CAD build for the part. Positions are in the model's coordinates, mm. A direction names the side the tool comes from. Give positions to 0.01 mm unless a question says otherwise; leave off trailing zeros. Order: outer loops, then holes, each group sorted by start corner. A loop starts at its lowest first (then second) coordinate and runs counter-clockwise, first axis right, second up.
```python
from build123d import *

# Parameters (mm, degrees)
BOSS_EXTRUDE1_DEPTH = 2
SKETCH2_R           = 0.74
CUT_EXTRUDE1_DEPTH  = 5.6
SKETCH6_W           = 79.5
SKETCH6_H           = 15
SKETCH6_R           = 3.2
CUT_EXTRUDE3_DEPTH  = 1.2
SKETCH7_R           = 3.2
SKETCH7_R_2         = 0.74
BOSS_EXTRUDE2_DEPTH = 1.4
SKETCH8_R           = 0.74
BOSS_EXTRUDE3_DEPTH = 0.4


with BuildPart() as part:
    # Sketch1 → Boss-Extrude1 (new body)
    with BuildSketch(Plane(origin=(0, 0, 0), x_dir=(1, 0, 0), z_dir=(0, 1, 0))):
        with BuildLine():
            ThreePointArc((7.5, 0), (5.303300859, -5.303300859), (0, -7.5))
            Line((0, -7.5), (72, -7.5))
            Line((72, -7.5), (72, 7.5))
            Line((72, 7.5), (0, 7.5))
            ThreePointArc((0, 7.5), (5.303300859, 5.303300859), (7.5, 0))
        make_face()
        with BuildLine():
            ThreePointArc((0, 7.5), (-7.5, 0), (0, -7.5))
            Line((0, -7.5), (0, 7.5))
        make_face()
        with BuildLine():
            Line((0, 7.5), (0, -7.5))
            ThreePointArc((0, -7.5), (5.303300859, -5.303300859), (7.5, 0))
            ThreePointArc((7.5, 0), (5.303300859, 5.303300859), (0, 7.5))
        make_face()
    extrude(amount=BOSS_EXTRUDE1_DEPTH)

    # Sketch2 → Cut-Extrude1 (cut)
    with BuildSketch(Plane(origin=(0, 2, 0), x_dir=(1, 0, 0), z_dir=(0, 1, 0))):
        Circle(SKETCH2_R)
    extrude(amount=-CUT_EXTRUDE1_DEPTH, mode=Mode.SUBTRACT)

    # Sketch6 → Cut-Extrude3 (cut)
    with BuildSketch(Plane(origin=(0, 2, 0), x_dir=(1, 0, 0), z_dir=(0, 1, 0))):
        with Locations((32.25, 0)):
            Rectangle(SKETCH6_W, SKETCH6_H)
        Circle(SKETCH6_R, mode=Mode.SUBTRACT)
    extrude(amount=-CUT_EXTRUDE3_DEPTH, mode=Mode.SUBTRACT)

    # Sketch7 → Boss-Extrude2 (add)
    with BuildSketch(Plane(origin=(0, 2, 0), x_dir=(1, 0, 0), z_dir=(0, 1, 0))):
        Circle(SKETCH7_R)
        Circle(SKETCH7_R_2, mode=Mode.SUBTRACT)
    extrude(amount=BOSS_EXTRUDE2_DEPTH)

    # Sketch8 → Boss-Extrude3 (add)
    with BuildSketch(Plane.XZ):
        Circle(SKETCH8_R)
    extrude(amount=-BOSS_EXTRUDE3_DEPTH)


solid = part.part
```
Item 1: Two-plate mould, pull along X, no slides. Class faces 1 (the face through (-7.5, 0.39, -0.16)), 2 (the face through (0, 0.4, 0)), 3 (the face through (32, 0.8, 0)): released by +X, released by -X, zero draft, split by the parting line, or undercut.
Item 2: Slice it at B-B (x = 33). Give the cut face in (y, z), and give its area (3 significant figures).
Item 3: Wall check: L1, parallel to X at y = 0.85, z = 0; L2, parallel to Y at x = 44, z = -0.5. Give the ranges that are in metal, low to high.
Item 4: Slice it at C-C (z = -5.75). Give the cut face in (x, y).
Item 5: Tool access for faces 4 (the face through (32, 0, 0)), 5 (the face through (-2.539, 2.118, 1.947)): list every direction of +Z, -Z, +X, -X, +Y, -Y with a clear straight run to the whole face (end or side of a thin tool).
Item 6: Drop flat-ended pins along their axis: pin 1 Ø5 at (x, z) = (7, -1) entering from +Y; pin 2 Ø1.6 at (x, z) = (0, 0) entering from +Y. Give the stop position or say it passes through.
Item 7: Slice it at A-A (z = 0). Give the cut face in (x, y).
A:
1. face 1: released by -X
1. face 2: undercut
1. face 3: zero draft
2. outline: (0, -7.5) - (0.8, -7.5) - (0.8, 7.5) - (0, 7.5) - close
2. area: 12.0 mm2
3. L1: x = -3.2 to -0.74, 0.74 to 3.2
3. L2: y = 0 to 0.8
4. outline: (-4.82, 0) - (72, 0) - (72, 0.8) - (-4.82, 0.8) - close
5. face 4: +Z, -Z, +X, -X, -Y
5. face 5: +Y
6. pin 1: stops at y = 0.8
6. pin 2: stops at y = 3.4
7. outline: (-7.5, 0) - (72, 0) - (72, 0.8) - (3.2, 0.8) - (3.2, 3.4) - (0.74, 3.4) - (0.74, 0.4) - (-0.74, 0.4) - (-0.74, 3.4) - (-3.2, 3.4) - (-3.2, 0.8) - (-7.5, 0.8) - close
